```python
from build123d import *

# Parameters (mm, degrees)
SKETCH1_R           = 0.5
BOSS_EXTRUDE1_DEPTH = 15.5
SKETCH1_3_R         = 1.2
BOSS_EXTRUDE2_DEPTH = 4.75
FILLET1_R           = 0.2
SKETCH2_R           = 0.85
BOSS_EXTRUDE3_DEPTH = 0.3
SKETCH4_W           = 0.461524445
SKETCH4_H           = 0.045344169
SKETCH7_W           = 0.600727217
SKETCH7_H           = 2.46


with BuildPart() as part:
    # Sketch1 → Boss-Extrude1 (new body)
    with BuildSketch(Plane.XY):
        Circle(SKETCH1_R)
    extrude(amount=BOSS_EXTRUDE1_DEPTH)



with BuildPart() as body_2:
    # Sketch1<3> → Boss-Extrude2 (new body)
    with BuildSketch(Plane.XY):
        Circle(SKETCH1_3_R)
    extrude(amount=-BOSS_EXTRUDE2_DEPTH)

    # Fillet1
    fillet1_edges = [body_2.edges().sort_by_distance(p)[0] for p in [
        (-1.2, 0, 0),
    ]]
    fillet(fillet1_edges, radius=FILLET1_R)


with BuildPart() as part_1:
    add(part.part)

    add(body_2.part)  # Boss-Extrude3 merges body 2
    # Sketch2 → Boss-Extrude3 (add)
    with BuildSketch(Plane.XY):
        Circle(SKETCH2_R)
    extrude(amount=BOSS_EXTRUDE3_DEPTH)

    # Sketch3 → Revolve1 (revolve)
    with BuildSketch(Plane(origin=(0, 0, 0), x_dir=(1, 0, 0), z_dir=(0, 1, 0))):
        with BuildLine():
            Line((0.5, -15.5), (0, -15.5))
            Line((0, -15.5), (0, -16.08))
            ThreePointArc((0, -16.08), (0.247487373, -16.182512627), (0.35, -16.43))
            Line((0.35, -16.43), (0.5, -16.43))
            ThreePointArc((0.5, -16.43), (0.430997893, -16.176542279), (0.243036734, -15.993041025))
            Line((0.243036734, -15.993041025), (0.243036734, -15.903342272))
            Line((0.243036734, -15.903342272), (0.447644951, -15.903342272))
            Line((0.447644951, -15.903342272), (0.447644951, -15.705896244))
            Line((0.447644951, -15.705896244), (0.36945341, -15.705896244))
            ThreePointArc((0.36945341, -15.705896244), (0.404840541, -15.583999079), (0.5, -15.5))
        make_face()
    revolve(axis=Axis((0, 0, 15.5), (0, 0, 1)))

    # Sketch4 → Revolve2 (revolve)
    with BuildSketch(Plane(origin=(0, 0, 0), x_dir=(1, 0, 0), z_dir=(0, 1, 0))):
        with Locations((-0.230762223, -16.317327916)):
            Rectangle(SKETCH4_W, SKETCH4_H)
    revolve(axis=Axis((0, 0, 15.5), (0, 0, 1)))

    # Sketch7 → Cut-Revolve1 (revolve, cut)
    with BuildSketch(Plane(origin=(0, 0, 0), x_dir=(1, 0, 0), z_dir=(0, 1, 0))):
        with Locations((-0.600363609, -14.27)):
            Rectangle(SKETCH7_W, SKETCH7_H)
    revolve(axis=Axis((0, 0, 15.5), (0, 0, 1)), mode=Mode.SUBTRACT)


solid = part_1.part
```
Read the model definition and answer for the solid it produces. Units are mm, in the model's axes. A direction names the side the tool comes from. Coordinates: 2 decimals unless noted, no trailing zeros. Write each loop counter-clockwise with the first axis right and the second up, starting at its lowest first coordinate (ties: lowest second). Pieces come first, ordered by that corner, then holes. Notation, with made-up numbers: (-8.5, 24) -> (0.5, 24) arc R23 cw to (0.5, 39) -> close; hole circle Ø7 at (43.25, 77.5). An arc over 180 degrees is marked (long way). Answer as a JSON object with one key per item and string values.
Q1. Flat-ended cylindrical pins translate along their axes: pin 1 Ø0.5 at (x, y) = (0, 0) entering from +Z; pin 2 Ø1 at (x, y) = (-1, -1) entering from +Z. Find the tip coordinate at first contact, or state that the pin passes through.
The answers:
{"pin 1": "stops at z = 16.34", "pin 2": "stops at z = 0"}
Q2. Consider line 1 (Z direction, x = 0.4, y = -0.85); line 2 (X direction, y = -0.05, z = 5.5); line 3 (Z direction, x = 0.5, y = -0.25). Determine where each line is inside the solid, lowest interval first. Write a range as [from, to].
The answers:
{"line 1": "z = [-4.75, 0]", "line 2": "x = [-0.5, 0.5]", "line 3": "z = [-4.75, 0.3]"}
Q3. The part is cut by section B-B on z = -2.5. Give the vertices of the cut face in (x, y), then the cut area to 3 significant figures.
The answers:
{"outline": "circle Ø2.4 at (0, 0)", "area": "4.52 mm2"}
Q4. The part is cut by section A-A on z = 12. Give the vertices of the cut face in (x, y), then the cut area to 3 significant figures.
The answers:
{"outline": "circle Ø1 at (0, 0)", "area": "0.785 mm2"}
Q5. A tool of negligible diameter and unlimited length cuts with its end or side. For faces 1 (the cylindrical face through (0.65, 1.01, -2.44)), 2 (the cylindrical face through (-0.108, -0.488, 6.581)), from which of +Z, -Z, +X, -X, +Y, -Y can it reach the whole face along a straight path? Write none if from no direction.
The answers:
{"face 1": "+Z, -Z", "face 2": "+Z"}
